Check sheet for the modelled part. Datum: model origin and axes. Units: mm. A direction names the side the tool comes from. Round coordinates to 2 decimals unless told otherwise and drop trailing zeros. Order: outer loops, then holes, each group sorted by start corner. A loop starts at its lowest first (then second) coordinate and runs counter-clockwise, first axis right, second up.
(1) Thickness scan on probe 1 along Z at (x, y) = (4.75, 33.5); probe 2 along X at (y, z) = (40, 0.45); probe 3 along Y at (x, z) = (-0.5, -10.25). Record the ranges inside material, lowest first.
(2) Mould release check, pull along Z, two halves, no side actions. Record for faces 4 (the flat face through (2, 40, -10.75)), 5 (the flat face through (8, 20, 2)), 6 (the flat face through (-3, 29, -5)): released by +Z, released by -Z, zero draft, split by the parting line, or undercut.
(3) Sectioned sample at A-A, the plane z = -12.25. Enter the section's corners in (x, y), and give its area (3 significant figures).
(4) Tool access check on faces 1 (the cylindrical face through (-0.715, -1.375, -8.299)), 2 (the flat face through (-3, 19, -5)), 3 (the cylindrical face through (-1.797, 21.126, -8.859)). Record the directions out of +Z, -Z, +X, -X, +Y, -Y that give a thin tool (end or side, any length) a straight path to the whole face; none if there is none.
(5) Sectioned sample at B-B, the plane y = 15. Enter the section's corners in (x, z).
(6) Sectioned sample at C-C, the plane y = 28. Count the separate pieces of the cut face and the enclosed holes in it, and give its area (3 significant figures).
(7) Depth check by flat-ended pin: pin 1 (3.5 mm diameter, centred on x = 0, y = 40, fed in from +Z); pin 2 (1.5 mm diameter, centred on x = 5.5, z = 2.5, fed in from -Y); pin 3 (1.5 mm diameter, centred on x = 6.5, z = 2.5, fed in from +Y); pin 4 (2 mm diameter, centred on x = 0, y = 0, fed in from +Z). Enter the tip coordinate at first touch or a pass-through.
```python
from build123d import *

# Parameters (mm, degrees)
SKETCH1_R           = 1.55
SKETCH1_R_2         = 1.25
BOSS_EXTRUDE1_DEPTH = 4.75
FILLET2_SIZE        = 1
SKETCH2_R           = 5
CUT_EXTRUDE1_DEPTH  = 4
SKETCH3_W           = 5
SKETCH3_H           = 18
BOSS_EXTRUDE2_DEPTH = 5
SKETCH8_R           = 4
SKETCH8_R_2         = 1.55
BOSS_EXTRUDE4_DEPTH = 4
FILLET3_R           = 4
SKETCH7_R           = 0.95
CUT_EXTRUDE3_DEPTH  = 53.423754158
CHAFL_N1_SIZE       = 0.25
CHAFL_N2_SIZE       = 3


with BuildPart() as part:
    # Sketch1 → Boss-Extrude1 (new body)
    with BuildSketch(Plane.XY):
        with BuildLine():
            Line((-8, 0), (-8, 40))
            ThreePointArc((-8, 40), (0, 48), (8, 40))
            Line((8, 40), (8, 0))
            ThreePointArc((8, 0), (0, -8), (-8, 0))
        make_face()
        with Locations((0, 40)):
            Circle(SKETCH1_R, mode=Mode.SUBTRACT)
        Circle(SKETCH1_R_2, mode=Mode.SUBTRACT)
    extrude(amount=BOSS_EXTRUDE1_DEPTH)

    # Fillet2
    fillet2_edges = [part.edges().sort_by_distance(p)[0] for p in [
        (0, 48, 4.75),
        (-8, 20, 4.75),
        (0, -8, 4.75),
        (8, 20, 4.75),
    ]]
    chamfer(fillet2_edges, length=FILLET2_SIZE)

    # Sketch2 → Cut-Extrude1 (cut)
    with BuildSketch(Plane.XY.offset(4.75)):
        with Locations((0, 40)):
            Circle(SKETCH2_R)
    extrude(amount=-CUT_EXTRUDE1_DEPTH, mode=Mode.SUBTRACT)

    # Sketch3 → Boss-Extrude2 (add)
    with BuildSketch(Plane(origin=(0, 0, 0), x_dir=(-1, 0, 0), z_dir=(0, 0, -1))):
        with Locations((5.5, 21)):
            Rectangle(SKETCH3_W, SKETCH3_H)
    extrude(amount=BOSS_EXTRUDE2_DEPTH)

    # Sketch8 → Boss-Extrude4 (add)
    with BuildSketch(Plane(origin=(0, 0, 0), x_dir=(-1, 0, 0), z_dir=(0, 0, -1))):
        with Locations(Location((0, 0, 0), (0, 0, 180))):
            Circle(SKETCH8_R)
        Circle(SKETCH8_R_2, mode=Mode.SUBTRACT)
    extrude(amount=BOSS_EXTRUDE4_DEPTH)

    # Fillet3
    fillet3_edges = [part.edges().sort_by_distance(p)[0] for p in [
        (-3, 21, 0),
    ]]
    fillet(fillet3_edges, radius=FILLET3_R)

    # Mirror5: part across plane


with BuildPart() as part_1:
    add(part.part)
    add(part.part.mirror(Plane.XY.offset(-5)))

    # Sketch7 → Cut-Extrude3 (cut, through all)
    with BuildSketch(Plane(origin=(0, 0, -14.75), x_dir=(-1, 0, 0), z_dir=(0, 0, -1))):
        with Locations((-3.5, 28)):
            Circle(SKETCH7_R)
        with Locations(Location((3.5, 28, 0), (0, 0, 180))):
            Circle(SKETCH7_R)
    extrude(amount=-CUT_EXTRUDE3_DEPTH, mode=Mode.SUBTRACT)

    # Chaflán1
    chafl_n1_edges = [part_1.edges().sort_by_distance(p)[0] for p in [
        (4.45, 28, 4.75),
        (4.45, 28, -14.75),
        (-4.45, 28, 4.75),
        (-4.45, 28, -14.75),
        (-1.25, 0, 4.75),
        (-5, 40, 4.75),
        (-5, 40, -14.75),
        (-1.25, 0, -14.75),
    ]]
    chamfer(chafl_n1_edges, length=CHAFL_N1_SIZE)

    # Chaflán2
    # the kernel refuses this chamfer: 3 mm, written as the material it takes off along each edge
    with BuildSketch(Plane(origin=(0, 0, -6), x_dir=(1, 0, 0), z_dir=(0, 1, 0))) as chafl_n2_piece_1:
        Polygon((4, CHAFL_N2_SIZE), (4 - CHAFL_N2_SIZE, 0), (4, 0), align=None)
    revolve(axis=Axis((0, 0, -6), (0, 0, -1)), mode=Mode.SUBTRACT)
    with BuildSketch(Plane(origin=(0, 0, -4), x_dir=(1, 0, 0), z_dir=(0, 1, 0))) as chafl_n2_piece_2:
        Polygon((4, -CHAFL_N2_SIZE), (4 - CHAFL_N2_SIZE, 0), (4, 0), align=None)
    revolve(axis=Axis((0, 0, -4), (0, 0, -1)), mode=Mode.SUBTRACT)


solid = part_1.part
```
Derived:
1. probe 1: z = -14.75 to -10, 0 to 4.75
1. probe 2: x = -8 to -1.55, 1.55 to 8
1. probe 3: y = -7.98 to -1.15, 1.15 to 38.53, 41.47 to 47.98
2. face 4: released by -Z
2. face 5: zero draft
2. face 6: undercut
3. outline: (-8, 0) arc R8 ccw to (8, 0) - (8, 40) arc R8 ccw to (-8, 40) - close; hole circle Ø10 at (0, 40); hole circle Ø1.9 at (-3.5, 28); hole circle Ø2.5 at (0, 0); hole circle Ø1.9 at (3.5, 28)
3. area: 752 mm2
4. face 1: none
4. face 2: +X, +Y, -Y
4. face 3: +X, +Y
5. outline: (-8, -13.75) - (-7, -14.75) - (7, -14.75) - (8, -13.75) - (8, -10) - (1, -10) arc R4 cw to (-3, -6) - (-3, -4) arc R4 cw to (1, 0) - (8, 0) - (8, 3.75) - (7, 4.75) - (-7, 4.75) - (-8, 3.75) - close
6. separate pieces: 5
6. enclosed holes: 0
6. area: 154 mm2
7. pin 1: stops at z = 0.75
7. pin 2: stops at y = -6.44
7. pin 3: stops at y = 45.56
7. pin 4: passes through
